Autodesk Inventor part; units mm, degrees
ref_plane "YZ Plane" through (0, 0, 0) normal (1, 0, 0) x (0, 1, 0)
ref_plane "XZ Plane" through (0, 0, 0) normal (0, 1, 0) x (-1, 0, 0)
ref_plane "XY Plane" through (0, 0, 0) normal (0, 0, 1) x (1, 0, 0)
sketch "スケッチ1" plane through (0, 0, 0) normal (0, 0, 1) x (1, 0, 0)
  line L0 (-2.5, 23.7333) -> (2.5, 23.7333)
  line L1 (2.5, 23.7333) -> (2.5, -36.2667)
  line L2 (2.5, -36.2667) -> (-2.5, -36.2667)
  line L3 (-2.5, -36.2667) -> (-2.5, 23.7333)
  point P0 (0, 0)
  dimension "d0" = 5
  dimension "d1" = 2.5
  dimension "d2" = 60
extrude "押し出し1" add sketch "スケッチ1" along normal blind 1
sketch "スケッチ2" plane through (0, 0, 1) normal (0, 0, 1) x (1, 0, 0)
  line L0 (2.5, 23.7333) -> (2.5, -36.2667)
  line L1 (-2.5, -36.2667) -> (2.5, -36.2667)
  line L2 (2.5, -36.2667) -> (2.5, -33.2667)
  line L3 (2.5, -33.2667) -> (-2.5, -33.2667)
  line L4 (-2.5, -33.2667) -> (-2.5, -36.2667)
  point P0 (0, 0)
  dimension "d5" = 3
extrude "押し出し2" cut sketch "スケッチ2" against normal blind 0.5
sketch "スケッチ4" plane through (0, 0, 0.5) normal (0, 0, 1) x (1, 0, 0)
  line L0 (2.5, -33.2667) -> (2.5, -36.2667)
  line L1 (2.5, -36.2667) -> (-2.5, -36.2667)
  line L2 (-3.5, -33.2667) -> (3.5, -33.2667)
  line L3 (3.5, -33.2667) -> (3.5, -36.2667)
  line L4 (3.5, -36.2667) -> (-3.5, -36.2667)
  line L5 (-3.5, -36.2667) -> (-3.5, -33.2667)
  point P0 (0, 0)
  dimension "d9" = 7
  dimension "d10" = 1
revolve "回転2" add sketch "スケッチ4" angle 360 about axis through (2.5, -36.2667, 0.5) along (-1, 0, 0)
fillet "フィレット1" radius 0.5 2 edges at (-3.5, -39.2667, 0.5) (3.5, -39.2667, 0.5)
properties part number "JointD2_2nd" material "アルミニウム 6061"
Read the model definition and answer for the solid it produces. Units are mm, in the model's axes. A direction names the side the tool comes from. Coordinates: 2 decimals unless noted, no trailing zeros. Loops run counter-clockwise (first coordinate to the right, second up) from the corner with the lowest first, then second, coordinate; pieces in that order, holes last.
Q1. Each of these flat-tipped pins is pushed along its axis until it touches: pin 1 Ø1 at (x, z) = (-0.5, 1.5) entering from -Y; pin 2 Ø3 at (x, z) = (-2, 3) entering from -Y; pin 3 Ø1.5 at (y, z) = (-1.5, 2) entering from -X; pin 4 Ø1 at (x, y) = (-1, 6) entering from +Z. Where does it stop, or does it pass through?
Q2. The part is cut by section A-A on x = -1.5. Write down the section's boundary in (y, z), and give its area (3 significant figures).
Q3. Which of the six approach directions +Z, -Z, +X, -X, +Y, -Y give full straight-line access (tool end or side, diameter ignored) to faces 1 (the face through (2.5, -4.4, 0.5)), 2 (the face through (-2.5, -5.2, 0.5)), 3 (the face through (-3.5, -36, 0)), 4 (the face through (0, -4, 1)), 5 (the face through (0, -4, 0))?
Q4. Consider probe 1 along Z at (x, y) = (-1.5, 2.5); probe 2 along X at (y, z) = (-18, 0.15); probe 3 along Y at (x, z) = (-3, -1.3). Determine where each line is inside the solid, lowest interval first.
Q5. The part is cut by section B-B on y = -28. Write down the section's boundary in (x, z).
Results below:
1. pin 1: stops at y = -39.22
1. pin 2: stops at y = -39.1
1. pin 3: passes through
1. pin 4: stops at z = 1
2. outline: (-33.31, 0) - (23.73, 0) - (23.73, 1) - (-33.27, 1) - (-33.27, 0.5) arc R3 ccw (long way) to start
2. area: 85.3 mm2
3. face 1: +Z, -Z, +X, +Y
3. face 2: +Z, -Z, -X, +Y
3. face 3: +Z, -Z, -X, +Y, -Y
3. face 4: +Z, +X, -X, +Y
3. face 5: -Z, +X, -X, +Y
4. probe 1: z = 0 to 1
4. probe 2: x = -2.5 to 2.5
4. probe 3: y = -38.67 to -33.87
5. outline: (-2.5, 0) - (2.5, 0) - (2.5, 1) - (-2.5, 1) - close
